Model file for the job. Use its own axes, mm. Coordinates: 2 decimals unless noted, no trailing zeros. Loops run counter-clockwise (first coordinate to the right, second up) from the corner with the lowest first, then second, coordinate; pieces in that order, holes last. Notation, with made-up numbers: M 57.25,32.5 L 62.25,32.5 A25 cw 62.25,55.5 Z; hole C 88.5,0 d6. An arc over 180 degrees is marked long. Write item = value, one per line. Start each with the question number.
from build123d import *

# Parameters (mm, degrees)
SKETCH1_W           = 220
SKETCH1_H           = 150
SKETCH1_W_2         = 3
SKETCH1_H_2         = 30
SKETCH1_W_3         = 30
SKETCH1_H_3         = 3
BOSS_EXTRUDE1_DEPTH = 3


with BuildPart() as part:
    # Sketch1 → Boss-Extrude1 (new body)
    with BuildSketch(Plane(origin=(0, 0, 0), x_dir=(1, 0, 0), z_dir=(0, 1, 0))):
        with Locations((110, 75)):
            Rectangle(SKETCH1_W, SKETCH1_H)
        with Locations((-1.5, 15)):
            Rectangle(SKETCH1_W_2, SKETCH1_H_2)
        with Locations((-1.5, 75)):
            Rectangle(SKETCH1_W_2, SKETCH1_H_2)
        with Locations((-1.5, 135)):
            Rectangle(SKETCH1_W_2, SKETCH1_H_2)
        with Locations((50, 151.5)):
            Rectangle(SKETCH1_W_3, SKETCH1_H_3)
        with Locations((110, 151.5)):
            Rectangle(SKETCH1_W_3, SKETCH1_H_3)
        with Locations((170, 151.5)):
            Rectangle(SKETCH1_W_3, SKETCH1_H_3)
        with Locations((221.5, 135)):
            Rectangle(SKETCH1_W_2, SKETCH1_H_2)
        with Locations((221.5, 75)):
            Rectangle(SKETCH1_W_2, SKETCH1_H_2)
        with Locations((221.5, 15)):
            Rectangle(SKETCH1_W_2, SKETCH1_H_2)
        with Locations((170, -1.5)):
            Rectangle(SKETCH1_W_3, SKETCH1_H_3)
        with Locations((110, -1.5)):
            Rectangle(SKETCH1_W_3, SKETCH1_H_3)
        with Locations((50, -1.5)):
            Rectangle(SKETCH1_W_3, SKETCH1_H_3)
    extrude(amount=BOSS_EXTRUDE1_DEPTH)


solid = part.part
Item 1: Pin check, flat tips, straight feed: pin 1 Ø1.5 at (y, z) = (1, -31) entering from +X; pin 2 Ø0.9 at (y, z) = (1.5, -151.5) entering from +X; pin 3 Ø0.9 at (x, y) = (203.5, 1.5) entering from +Z. Stop position of each tip, or through.
Item 2: Cut at B-B (z = -48). Give the cut face in (x, y).
Item 3: Probe L1, parallel to X at y = 0.85, z = -52; L2, parallel to Z at x = 17, y = 2.25. List the from-to ranges inside material, lowest first.
Item 4: Cut at A-A (x = 89). Give the cut face in (y, z).
Reported:
q1.pin_1 = 220
q1.pin_2 = 185
q1.pin_3 = 0
q2.outline = M 0,0 L 220,0 L 220,3 L 0,3 Z
q3.L1 = 0 to 220
q3.L2 = -150 to 0
q4.outline = M 0,-150 L 3,-150 L 3,0 L 0,0 Z
